Model file for the job. Use its own axes, mm. A direction names the side the tool comes from. Coordinates: 2 decimals unless noted, no trailing zeros. Order: outer loops, then holes, each group sorted by start corner. A loop starts at its lowest first (then second) coordinate and runs counter-clockwise, first axis right, second up.
from build123d import *

# Parameters (mm, degrees)
EXTRUDE_1_DEPTH     = 5
FILLET_1_R          = 2
SKETCH_2_R          = 4.25
CUT_EXTRUDE_1_DEPTH = 90.582364336


with BuildPart() as part:
    # 草图1 → 凸台-拉伸1 (new body)
    with BuildSketch(Plane.XY):
        Polygon((17.5, 17.5), (80, 17.5), (80, -17.5), (17.5, -17.5), (17.5, -40), (-17.5, -40), (-17.5, -17.5), (-80, -17.5), (-80, 17.5), (-17.5, 17.5), (-17.5, 40), (17.5, 40), align=None)
    extrude(amount=EXTRUDE_1_DEPTH)

    # 圆角1
    fillet_1_edges = [part.edges().sort_by_distance(p)[0] for p in [
        (80, -17.5, 2.5),
        (17.5, -40, 2.5),
        (-17.5, -40, 2.5),
        (-80, -17.5, 2.5),
        (-80, 17.5, 2.5),
        (-17.5, 40, 2.5),
        (17.5, 40, 2.5),
        (80, 17.5, 2.5),
    ]]
    fillet(fillet_1_edges, radius=FILLET_1_R)

    # 草图2 → 切除-拉伸1 (cut, through all)
    with BuildSketch(Plane.XY.offset(5)):
        with Locations((0, 30)):
            Circle(SKETCH_2_R)
        with Locations((-65.712823547, 0)):
            Circle(SKETCH_2_R)
        with Locations((-30.923378323, 0)):
            Circle(SKETCH_2_R)
    cut_extrude_1 = extrude(amount=-CUT_EXTRUDE_1_DEPTH, mode=Mode.SUBTRACT)

    # 镜向1: 切除-拉伸1 across plane
    add(cut_extrude_1.mirror(Plane.ZX), mode=Mode.SUBTRACT)

    # 镜向2: 切除-拉伸1 across plane
    add(cut_extrude_1.mirror(Plane(origin=(0, 0, 0), x_dir=(0, 0, 1), z_dir=(1, 0, 0))), mode=Mode.SUBTRACT)


solid = part.part
Q1. Cut at D-D, the plane z = 3.1. List the corners of the cut face in (x, y), plus the area to 3 significant figures.
Established:
outline: (-80, -15.5) arc R2 ccw to (-78, -17.5) - (-17.5, -17.5) - (-17.5, -38) arc R2 ccw to (-15.5, -40) - (15.5, -40) arc R2 ccw to (17.5, -38) - (17.5, -17.5) - (78, -17.5) arc R2 ccw to (80, -15.5) - (80, 15.5) arc R2 ccw to (78, 17.5) - (17.5, 17.5) - (17.5, 38) arc R2 ccw to (15.5, 40) - (-15.5, 40) arc R2 ccw to (-17.5, 38) - (-17.5, 17.5) - (-78, 17.5) arc R2 ccw to (-80, 15.5) - close; hole circle Ø8.5 at (-65.71, 0); hole circle Ø8.5 at (-30.92, 0); hole circle Ø8.5 at (0, -30); hole circle Ø8.5 at (0, 30); hole circle Ø8.5 at (30.92, 0); hole circle Ø8.5 at (65.71, 0)
area: 6,830 mm2
Q2. Cut at B-B, the plane y = 0. List the corners of the cut face in (x, z).
Established:
outline: (-80, 0) - (-69.96, 0) - (-69.96, 5) - (-80, 5) - close; (-61.46, 0) - (-35.17, 0) - (-35.17, 5) - (-61.46, 5) - close; (-26.67, 0) - (26.67, 0) - (26.67, 5) - (-26.67, 5) - close; (35.17, 0) - (61.46, 0) - (61.46, 5) - (35.17, 5) - close; (69.96, 0) - (80, 0) - (80, 5) - (69.96, 5) - close
Q3. Cut at C-C, the plane y = 30. List the corners of the cut face in (x, z).
Established:
outline: (-17.5, 0) - (-4.25, 0) - (-4.25, 5) - (-17.5, 5) - close; (4.25, 0) - (17.5, 0) - (17.5, 5) - (4.25, 5) - close
Q4. Cut at A-A, the plane x = 0. List the corners of the cut face in (y, z).
Established:
outline: (-40, 0) - (-34.25, 0) - (-34.25, 5) - (-40, 5) - close; (-25.75, 0) - (25.75, 0) - (25.75, 5) - (-25.75, 5) - close; (34.25, 0) - (40, 0) - (40, 5) - (34.25, 5) - close
Q5. Which spindle directions (+Z, -Z, +X, -X, +Y, -Y) get a long thin tool onto all of the face, cutting with end or side? Do faces 4 (the face through (-66.266, 4.214, 2.535)), 5 (the face through (-47, -17.5, 2)), 6 (the face through (47, 17.5, 2)), 7 (the face through (-48, 17.5, 2)). Say none if no direction does.
Established:
face 4: +Z, -Z
face 5: +Z, -Z, -X, -Y
face 6: +Z, -Z, +X, +Y
face 7: +Z, -Z, -X, +Y
Q6. Drop flat-ended pins along their axis: P1, Ø10, axis at x = 30.92, y = 0, coming from the +Z side; P2, Ø1.5, axis at y = 29, z = 2.5, coming from the -X side; P3, Ø2.5, axis at x = 48, z = 3, coming from the -Y side; P4, Ø2.5, axis at x = 32.5, z = 2.5, coming from the +Y side. Give the stop position or say it passes through.
Established:
P1: stops at z = 5
P2: stops at x = -17.5
P3: stops at y = -17.5
P4: stops at y = 17.5
Q7. Mould opens along Y. For faces 1 (the face through (48, -17.5, 2)), 2 (the face through (-26.87, 1.28, 2.54)), 3 (the face through (-17.5, -28, 2)) say: pulls with the +Y half, pulls with the -Y half, needs draft (parallel to the pull), parting line crosses it, or undercut.
Established:
face 1: pulls with the -Y half
face 2: undercut
face 3: needs draft
Q8. Probe line 1 (Y direction, x = 3.5, z = 0.75); line 2 (X direction, y = -27.5, z = 1.45); line 3 (X direction, y = 35, z = 1.3). List the from-to ranges inside material, lowest first.
Established:
line 1: y = -40 to -32.41, -27.59 to 27.59, 32.41 to 40
line 2: x = -17.5 to -3.44, 3.44 to 17.5
line 3: x = -17.5 to 17.5
